Design review of the part built by this model. Coordinates are the model's own, in mm. Face numbers are marked on the shaded views. Coordinates: 2 decimals unless noted, no trailing zeros. Loops run counter-clockwise (first coordinate to the right, second up) from the corner with the lowest first, then second, coordinate; pieces in that order, holes last. Notation, with made-up numbers: (-6.5, 47) -> (13.5, 47) arc R19 cw to (13.5, 66) -> close; hole circle Ø10 at (69, 65.25). An arc over 180 degrees is marked (long way). Use CSV: the item, a comma, the result in double quotes.
```python
from build123d import *

# Parameters (mm, degrees)
SKETCH1_R           = 4
BOSS_EXTRUDE1_DEPTH = 6
CHAMFER1_SIZE       = 1


with BuildPart() as part:
    # Sketch1 → Boss-Extrude1 (new body)
    with BuildSketch(Plane(origin=(0, 0, 0), x_dir=(1, 0, 0), z_dir=(0, 1, 0))):
        Polygon((6.781243349, -4.398644334), (7.19995941, 3.673406842), (0.418716061, 8.072051176), (-6.781243349, 4.398644334), (-7.19995941, -3.673406842), (-0.418716061, -8.072051176), align=None)
        with Locations(Location((0, 0, 0), (0, 0, 270))):  # turned: the seam where the file's is
            Circle(SKETCH1_R, mode=Mode.SUBTRACT)
    extrude(amount=BOSS_EXTRUDE1_DEPTH)

    # Chamfer1
    chamfer1_edges = [part.edges().sort_by_distance(p)[0] for p in [
        (3.809337736, 6, -5.872729009),
        (-3.181263644, 6, -6.235347755),
        (-6.990601379, 6, -0.362618746),
        (0, 0, -4),
        (0, 6, -4),
        (-3.809337736, 6, 5.872729009),
        (3.181263644, 6, 6.235347755),
        (-3.809337736, 0, 5.872729009),
        (-6.990601379, 0, -0.362618746),
        (-3.181263644, 0, -6.235347755),
        (6.990601379, 6, 0.362618746),
        (3.809337736, 0, -5.872729009),
        (6.990601379, 0, 0.362618746),
        (3.181263644, 0, 6.235347755),
    ]]
    chamfer(chamfer1_edges, length=CHAMFER1_SIZE)


solid = part.part
```
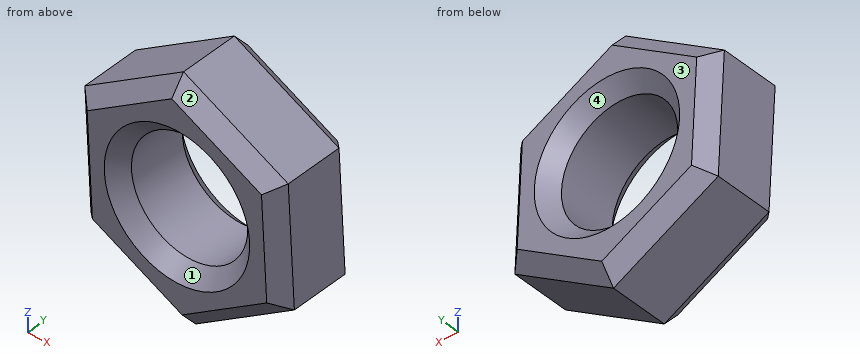
Item 1: Add section C-C (y = 5.5). Give the boundary of the cut face in (x, z), then the cut area to 3 significant figures.
Checked values:
outline,"(-6.69, 3.41) -> (-6.3, -4.08) -> (0.39, -7.5) -> (6.69, -3.41) -> (6.3, 4.08) -> (-0.39, 7.5) -> close; hole circle Ø9 at (0, 0)"
area,"82.7 mm^2"
Item 2: To check wall thickness, follow line 1 along X through (y, z) = (4, -1); line 2 along X through (y, z) = (2.3, 0); line 3 along Z through (x, y) = (-1, 4) (3 decimals). State the ranges of each line that lie inside material, in increasing order.
Checked values:
line 1,"-6.96 to -3.87, 3.87 to 7.06"
line 2,"-7.01 to -4, 4 to 7.01"
line 3,"-7.348 to -3.873, 3.873 to 7.695"
Item 3: Clearance check with flat-ended pins moving along their axes: pin 1 (1 mm diameter, centred on x = -1.5, z = 0.5, fed in from -Y); pin 2 (3 mm diameter, centred on x = 2.5, y = 2.5, fed in from +Z). State where each tip first meets the part, or that it passes through.
Checked values:
pin 1,"through"
pin 2,"z = 7.35"
Item 4: Draft analysis for pull direction X (two halves, no side actions). For the marked faces 1, 2, 3 and 4, state which applies: pulls with the +X half, pulls with the -X half, needs draft (parallel to the pull), parting line crosses it, or undercut.
Checked values:
face 1,"undercut"
face 2,"pulls with the +X half"
face 3,"needs draft"
face 4,"undercut"
Item 5: Add section B-B (z = 0). Give the boundary of the cut face in (x, y).
Checked values:
outline,"(-7.01, 1) -> (-6.01, 0) -> (-5, 0) -> (-4, 1) -> (-4, 5) -> (-5, 6) -> (-6.01, 6) -> (-7.01, 5) -> close; (4, 1) -> (5, 0) -> (6.01, 0) -> (7.01, 1) -> (7.01, 5) -> (6.01, 6) -> (5, 6) -> (4, 5) -> close"
Item 6: Add section D-D (z = 6.25). Give the boundary of the cut face in (x, y).
Checked values:
outline,"(-3.23, 1) -> (-1.39, 0) -> (0.95, 0) -> (3.15, 1) -> (3.15, 5) -> (0.95, 6) -> (-1.39, 6) -> (-3.23, 5) -> close"
Item 7: Add section A-A (x = 0). Give the boundary of the cut face in (y, z).
Checked values:
outline,"(0, -6.74) -> (1, -7.86) -> (5, -7.86) -> (6, -6.74) -> (6, -5) -> (5, -4) -> (1, -4) -> (0, -5) -> close; (0, 5) -> (1, 4) -> (5, 4) -> (6, 5) -> (6, 6.74) -> (5, 7.86) -> (1, 7.86) -> (0, 6.74) -> close"
